```python
from build123d import *

# Parameters (mm, degrees)
SKETCH13_R          = 20
CUT_EXTRUDE1_DEPTH  = 29
SKETCH14_R          = 11.397429613
BOSS_EXTRUDE1_DEPTH = 25


with BuildPart() as part:
    # Sketch12 → Revolve2 (revolve)
    with BuildSketch(Plane.XY, mode=Mode.PRIVATE) as revolve2_sk:
        with BuildLine():
            Line((1.036180374, -5.869273447), (5, -28.321678322))
            Line((5, -28.321678322), (5, -65))
            ThreePointArc((5, -65), (6.464466094, -68.535533906), (10, -70))
            Line((10, -70), (30, -70))
            Line((30, -70), (30, 0))
            Line((30, 0), (5.960036959, 0))
            ThreePointArc((5.960036959, 0), (2.129477781, -1.786463571), (1.036180374, -5.869273447))
        make_face()
    revolve(revolve2_sk.sketch.rotate(Axis((30, -70, 0), (0, 1, 0)), 270), axis=Axis((30, -70, 0), (0, 1, 0)))

    # Sketch13 → Cut-Extrude1 (cut)
    with BuildSketch(Plane(origin=(0, 0, 0), x_dir=(1, 0, 0), z_dir=(0, 1, 0))):
        with Locations(Location((29.644688486, 0, 0), (0, 0, 270))):
            Circle(SKETCH13_R)
    extrude(amount=-CUT_EXTRUDE1_DEPTH, mode=Mode.SUBTRACT)

    # Sketch14 → Boss-Extrude1 (add)
    with BuildSketch(Plane.XY):
        with Locations((28.772395524, -45.877146633)):
            Circle(SKETCH14_R)
    extrude(amount=BOSS_EXTRUDE1_DEPTH)


solid = part.part
```
The listing builds one solid part. Answer for the finished solid, in the listing's coordinates (mm). A direction names the side the tool comes from. Round coordinates to 2 decimals unless told otherwise and drop trailing zeros. Order: outer loops, then holes, each group sorted by start corner. A loop starts at its lowest first (then second) coordinate and runs counter-clockwise, first axis right, second up. Notation, with made-up numbers: (-38.5, -20) - (-6.5, -20) arc R10 ccw to (-6.5, -5) - close; hole circle Ø8 at (38, 30). An arc over 180 degrees is marked (long way). Put each result on its own line as item: value. Start each with the question number.
(1) Given P1, Ø4, axis at x = 10.5, y = -38.5, coming from the +Z side; P2, Ø1, axis at y = -40.5, z = -20, coming from the -X side; P3, Ø8, axis at x = 16.5, y = -33.5, coming from the +Z side, each flat-ended and moving along its own axis, determine where each tip first touches the part or whether it passes through.
(2) Determine the mould class of faces 1 (the conical face through (53.132, -22.242, -12.031)), 2 (the flat face through (49.5, 0, -3.7)), 3 (the flat face through (30, -29, 0)) for opening direction Z: released by +Z, released by -Z, zero draft, split by the parting line, or undercut.
(3) Find section C-C (y = -14.5). Give the vertices of the cut face in (x, z), plus the area to 3 significant figures.
(4) Find section A-A (z = 0). Give the vertices of the cut face in (x, y).
(5) For faces 4 (the flat face through (30, -70, 0)), 5 (the cylindrical face through (46.51, -14.3, 10.75)), 6 (the flat face through (29, -46, 25)), determine the directions among +Z, -Z, +X, -X, +Y, -Y from which every point of the face is accessible in a straight line to the end or side of a thin tool.
(6) Straight lines are drawn through the part: probe 1 along X at (y, z) = (-19.25, 0); probe 2 along X at (y, z) = (-9.5, 0); probe 3 along X at (y, z) = (-55.5, 1). For each, find the intervals that lie inside material, in ascending order. Write a range as from..to.
(7) Find section B-B (y = -32.5). Give the vertices of the cut face in (x, z), plus the area to 3 significant figures.
(8) Find section D-D (y = -55). Give the vertices of the cut face in (x, z).
Reply:
1. P1: z = 17.85
1. P2: x = 14.36
1. P3: z = 23.12
2. face 1: split by the parting line
2. face 2: zero draft
2. face 3: undercut
3. outline: circle Ø54.88 at (30, 0); hole circle Ø40 at (29.64, 0)
3. area: 1,110 mm^2
4. outline: (1.04, -5.87) - (5, -28.32) - (5, -65) arc R5 ccw to (10, -70) - (50, -70) arc R5 ccw to (55, -65) - (55, -28.32) - (58.96, -5.87) arc R5 ccw to (54.04, 0) - (49.64, 0) - (49.64, -29) - (9.64, -29) - (9.64, 0) - (5.96, 0) arc R5 ccw to start
5. face 4: +Z, -Z, +X, -X, -Y
5. face 5: +Y
5. face 6: +Z, +X, -X, -Y
6. probe 1: 3.4..9.64, 49.64..56.6
6. probe 2: 1.68..9.64, 49.64..58.32
6. probe 3: 5.02..54.98
7. outline: circle Ø50 at (30, 0)
7. area: 1,960 mm^2
8. outline: (21.94, 23.67) arc R25 ccw (long way) to (35.6, 24.36) - (35.6, 25) - (21.94, 25) - close
